Can you work these out from the model? Positions are in its coordinate system, mm. A direction names the side the tool comes from. Give positions to 0.01 mm unless a question says otherwise; leave off trailing zeros. Loops run counter-clockwise (first coordinate to the right, second up) from the corner with the lowest first, then second, coordinate; pieces in that order, holes last. Notation, with made-up numbers: (74.5, 5.5) - (133.5, 5.5) arc R31 ccw to (133.5, 34.5) - close; hole circle Ø3 at (34, 11). An arc over 180 degrees is marked (long way). Write item = value, one per line.
from build123d import *

# Parameters (mm, degrees)
F0_W     = 50.8
F0_H     = 19.05
F1_DEPTH = 774.7
F2_W     = 122.43557321
F2_H     = 50.8
F2_W_2   = 343.1604206562
F3_DEPTH = 25.4
F4_R     = 0.79375
F5_DEPTH = 25.4
F6_R     = 4.7625
F7_DEPTH = 25.4


# Not quite as in the source:
# - a feature names something its author has since deleted; it is built from what else it names


with BuildPart() as f1:
    # F0 (on Top) → F1 (new body)
    with BuildSketch(Plane.XY):
        Rectangle(F0_W, F0_H)
    extrude(amount=F1_DEPTH)

    # F2 (on Front) → F3 (cut)
    with BuildSketch(Plane.XZ):
        with Locations((22.4465244144, 25.4)):
            Rectangle(F2_W, F2_H)
        with Locations((-38.7818217278, 749.3)):
            Rectangle(F2_W_2, F2_H)
    extrude(amount=F3_DEPTH, mode=Mode.SUBTRACT)

    # F4 (on Front) → F5 (cut)
    with BuildSketch(Plane.XZ):
        with Locations((9.525, 101.6)):
            Circle(F4_R)
        with Locations((9.525, 155.575)):
            Circle(F4_R)
        with Locations((9.525, 619.125)):
            Circle(F4_R)
        with Locations((9.525, 673.1)):
            Circle(F4_R)
        with Locations((-9.525, 619.125)):
            Circle(F4_R)
        with Locations((-9.525, 673.1)):
            Circle(F4_R)
        with Locations((-9.525, 101.6)):
            Circle(F4_R)
        with Locations((-9.525, 155.575)):
            Circle(F4_R)
    extrude(amount=-F5_DEPTH, mode=Mode.SUBTRACT)

    # F6 (on Front) → F7 (cut)
    with BuildSketch(Plane.XZ):
        with Locations((-15.875, 361.95)):
            Circle(F6_R)
    extrude(amount=F7_DEPTH, mode=Mode.SUBTRACT)


solid = f1.part
Q1. Imagine slicing it at A-A, the plane x = 2.5. Write out the boundary of the cut face in (y, z) (3 decimals), then the cut area to 3 significant figures.
Output:
outline = (-9.525, 50.8) - (0, 50.8) - (0, 0) - (9.525, 0) - (9.525, 774.7) - (0, 774.7) - (0, 723.9) - (-9.525, 723.9) - close
area = 13,800 mm2
Q2. I need wall thicknesses on L1, parallel to X at y = 5.75, z = 101.6; L2, parallel to Z at x = -5, y = -7.75; L3, parallel to Y at x = 11.5, z = 46.5 (3 decimals). Which ranges of each line are inside material? Lowest first, please.
Output:
L1 = -25.4 to -10.32, -8.73 to 8.73, 10.32 to 25.4
L2 = 50.8 to 723.9
L3 = 0 to 9.525
Q3. Which directions (+Z, -Z, +X, -X, +Y, -Y) give clear straight access to the entire face, cutting with the end or side of a thin tool? Please do faces 1 (the flat face through (-25.4, 0, 382)), 2 (the flat face through (0, 0, 26)), 3 (the flat face through (0, 0, 750)).
Output:
face_1 = +Z, -Z, -X, +Y, -Y
face_2 = -Z, +X, -X, -Y
face_3 = +Z, +X, -X, -Y
Q4. For pin 1 (5 mm diameter, centred on x = -7, y = -4.5, fed in from -Z); pin 2 (1 mm diameter, centred on x = -9.525, z = 619.125, fed in from +Y), each with a flat end and sliding along its axis, tell me the tip position at first contact or that it passes through.
Output:
pin_1 = 50.8
pin_2 = 0
